The listing builds one solid part. Answer for the finished solid, in the listing's coordinates (mm). Face numbers are marked on the shaded views. A direction names the side the tool comes from. Round coordinates to 2 decimals unless told otherwise and drop trailing zeros. Write each loop counter-clockwise with the first axis right and the second up, starting at its lowest first coordinate (ties: lowest second). Pieces come first, ordered by that corner, then holes.
(1) Each of these flat-tipped pins is pushed along its axis until it touches: pin 1 Ø12.5 at (y, z) = (17, 15.5) entering from +X; pin 2 Ø0.5 at (x, y) = (-59.5, 54.5) entering from +Z; pin 3 Ø3 at (x, z) = (-59.5, 24) entering from -Y. Where does it stop, or does it pass through?
(2) For the marked faces 4, 5, 6 and 7, determine the directions among +Z, -Z, +X, -X, +Y, -Y from which every point of the face is accessible in a straight line to the end or side of a thin tool.
(3) A cutting plane is placed at A-A, the plane z = 20. Give the vertices of the cut face in (x, y).
(4) A cutting plane is placed at B-B, the plane y = 2.4. Give the vertices of the cut face in (x, z), and give its area (3 significant figures).
(5) Find the intervals of material crossed by probe 1 along X at (y, z) = (51, 22.5); probe 2 along Z at (x, y) = (-4, -8); probe 3 along Y at (x, z) = (-44.5, 24.25), in increasing order.
(6) A cutting plane is placed at D-D, the plane y = 75.5. Give the vertices of the cut face in (x, z).
(7) The mould has two halves that part along Y. Classify the marked faces 1, 2 and 3: +Y half, -Y half, draft (parallel to the pull), parting line (faces both ways), or undercut.
(8) A cutting plane is placed at C-C, the plane x = -30. Give the vertices of the cut face in (y, z).
from build123d import *

# Parameters (mm, degrees)
F1_DEPTH = 25
F3_DEPTH = 2.5
F5_DEPTH = 5.2


with BuildPart() as f1:
    # F0 (on Top) → F1 (new body)
    with BuildSketch(Plane.XY):
        with BuildLine():
            Line((-1, 0), (0, 0))
            Line((0, 0), (0, 56))
            ThreePointArc((0, 56), (-30, 86), (-60, 56))
            Line((-60, 56), (-60, 0))
            Line((-60, 0), (-59, 0))
            Line((-59, 0), (-59, 56))
            ThreePointArc((-59, 56), (-30, 85), (-1, 56))
            Line((-1, 56), (-1, 0))
        make_face()
        with BuildLine():
            ThreePointArc((-60, 0), (-30, -30), (0, 0))
            Line((0, 0), (-1, 0))
            ThreePointArc((-1, 0), (-30, -29), (-59, 0))
            Line((-59, 0), (-60, 0))
        make_face()
    extrude(amount=F1_DEPTH)

    # F2 (on face) → F3 (join)
    with BuildSketch(Plane.XY.offset(25)):
        with BuildLine():
            ThreePointArc((2.5, 56), (-30, 88.5), (-62.5, 56))
            Line((-62.5, 56), (-62.5, 0))
            ThreePointArc((-62.5, 0), (-30, -32.5), (2.5, 0))
            Line((2.5, 0), (2.5, 56))
        make_face()
        with BuildLine():
            Line((-60, 0), (-60, 56))
            ThreePointArc((-60, 56), (-30, 86), (0, 56))
            Line((0, 56), (0, 0))
            ThreePointArc((0, 0), (-30, -30), (-60, 0))
        make_face(mode=Mode.SUBTRACT)
        with BuildLine():
            ThreePointArc((0, 56), (-30, 86), (-60, 56))
            Line((-60, 56), (-60, 0))
            ThreePointArc((-60, 0), (-30, -30), (0, 0))
            Line((0, 0), (0, 56))
        make_face()
        with BuildLine():
            ThreePointArc((-1, 0), (-30, -29), (-59, 0))
            Line((-59, 0), (-59, 56))
            ThreePointArc((-59, 56), (-30, 85), (-1, 56))
            Line((-1, 56), (-1, 0))
        make_face(mode=Mode.SUBTRACT)
        with BuildLine():
            Line((-59, 56), (-59, 0))
            ThreePointArc((-59, 0), (-30, -29), (-1, 0))
            Line((-1, 0), (-1, 56))
            ThreePointArc((-1, 56), (-30, 85), (-59, 56))
        make_face()
    extrude(amount=F3_DEPTH)

    # F4 (on face) → F5 (cut)
    with BuildSketch(Plane.XY.offset(27.5)):
        with BuildLine():
            Line((-58.5, 56), (-62.5, 56))
            Line((-62.5, 56), (-62.5, 51.2))
            Line((-62.5, 51.2), (-58.5, 51.2))
            ThreePointArc((-58.5, 51.2), (-56.1, 53.6), (-58.5, 56))
        make_face()
        with BuildLine():
            Line((-58.5, 4.8), (-62.5, 4.8))
            Line((-62.5, 4.8), (-62.5, 0))
            Line((-62.5, 0), (-58.5, 0))
            ThreePointArc((-58.5, 0), (-56.1, 2.4), (-58.5, 4.8))
        make_face()
    extrude(amount=-F5_DEPTH, mode=Mode.SUBTRACT)


solid = f1.part
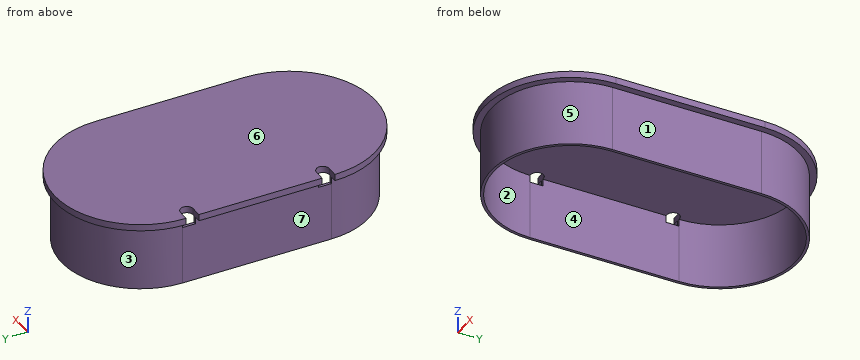
Solutions:
1. pin 1: stops at x = 0
1. pin 2: stops at z = 22.3
1. pin 3: stops at y = -15.83
2. face 4: -Z
2. face 5: -Z, -Y
2. face 6: +Z, +X, -X, +Y, -Y
2. face 7: -Z, -X, +Y, -Y
3. outline: (-60, 0) arc R30 ccw to (0, 0) - (0, 56) arc R30 ccw to (-60, 56) - close; hole (-59, 0) arc R29 ccw to (-1, 0) - (-1, 56) arc R29 ccw to (-59, 56) - close
4. outline: (-60, 0) - (-59, 0) - (-59, 22.3) - (-60, 22.3) - close; (-56.1, 25) - (-1, 25) - (-1, 0) - (0, 0) - (0, 25) - (2.5, 25) - (2.5, 27.5) - (-56.1, 27.5) - close
4. area: 194 mm2
5. probe 1: x = -60 to -59, -1 to 0
5. probe 2: z = 25 to 27.5
5. probe 3: y = -26.26 to -25.11, 81.11 to 82.26
6. outline: (-56, 25) - (-52.8, 25) - (-52.8, 0) - (-51.47, 0) - (-51.47, 25) - (-8.53, 25) - (-8.53, 0) - (-7.2, 0) - (-7.2, 25) - (-4, 25) - (-4, 27.5) - (-56, 27.5) - close
7. face 1: draft
7. face 2: undercut
7. face 3: +Y half
8. outline: (-32.5, 25) - (-30, 25) - (-30, 0) - (-29, 0) - (-29, 25) - (85, 25) - (85, 0) - (86, 0) - (86, 25) - (88.5, 25) - (88.5, 27.5) - (-32.5, 27.5) - close
